```python
from build123d import *

# Parameters (mm, degrees)
BOSS_EXTRUDE1_DEPTH      = 2
CIRPATTERN1_COUNT        = 11
BOSS_EXTRUDE2_DEPTH      = 2
BOSS_EXTRUDE2_DEPTH_BACK = 2
SKETCH4_R                = 17.5
SKETCH6_R                = 14.669
SKETCH6_R_2              = 12.669
BOSS_EXTRUDE4_DEPTH      = 0.5
SKETCH7_R                = 10
CUT_EXTRUDE1_DEPTH       = 4
SKETCH8_W                = 2
SKETCH8_H                = 1.2
BOSS_EXTRUDE5_DEPTH      = 4
CIRPATTERN2_COUNT        = 12


with BuildPart() as part:
    # Sketch2 → Boss-Extrude1 (new, symmetric)
    with BuildSketch(Plane.XY):
        with BuildLine():
            Line((-0.5, 23.626113967), (0.5, 23.626113967))
            ThreePointArc((0.5, 23.626113967), (1.603484659, 21.216683922), (2.671054487, 18.791127038))
            ThreePointArc((2.671054487, 18.791127038), (3.577591086, 17.539110484), (4.930319745, 16.791127038))
            ThreePointArc((4.930319745, 16.791127038), (0, 17.5), (-4.930319745, 16.791127038))
            ThreePointArc((-4.930319745, 16.791127038), (-3.577591086, 17.539110484), (-2.671054487, 18.791127038))
            ThreePointArc((-2.671054487, 18.791127038), (-1.603484659, 21.216683922), (-0.5, 23.626113967))
        make_face()
    extrude(amount=BOSS_EXTRUDE1_DEPTH, both=True)


with BuildPart() as cirpattern1_1:
    # CirPattern1: pattern copy
    add(part.part.rotate(Axis((0, 0, 0), (0, 0, 1)), 1 * 360 / CIRPATTERN1_COUNT))


with BuildPart() as cirpattern1_2:
    # CirPattern1: pattern copy
    add(part.part.rotate(Axis((0, 0, 0), (0, 0, 1)), 2 * 360 / CIRPATTERN1_COUNT))


with BuildPart() as cirpattern1_3:
    # CirPattern1: pattern copy
    add(part.part.rotate(Axis((0, 0, 0), (0, 0, 1)), 3 * 360 / CIRPATTERN1_COUNT))


with BuildPart() as cirpattern1_4:
    # CirPattern1: pattern copy
    add(part.part.rotate(Axis((0, 0, 0), (0, 0, 1)), 4 * 360 / CIRPATTERN1_COUNT))


with BuildPart() as cirpattern1_5:
    # CirPattern1: pattern copy
    add(part.part.rotate(Axis((0, 0, 0), (0, 0, 1)), 5 * 360 / CIRPATTERN1_COUNT))


with BuildPart() as cirpattern1_6:
    # CirPattern1: pattern copy
    add(part.part.rotate(Axis((0, 0, 0), (0, 0, 1)), 6 * 360 / CIRPATTERN1_COUNT))


with BuildPart() as cirpattern1_7:
    # CirPattern1: pattern copy
    add(part.part.rotate(Axis((0, 0, 0), (0, 0, 1)), 7 * 360 / CIRPATTERN1_COUNT))


with BuildPart() as cirpattern1_8:
    # CirPattern1: pattern copy
    add(part.part.rotate(Axis((0, 0, 0), (0, 0, 1)), 8 * 360 / CIRPATTERN1_COUNT))


with BuildPart() as cirpattern1_9:
    # CirPattern1: pattern copy
    add(part.part.rotate(Axis((0, 0, 0), (0, 0, 1)), 9 * 360 / CIRPATTERN1_COUNT))


with BuildPart() as cirpattern1_10:
    # CirPattern1: pattern copy
    add(part.part.rotate(Axis((0, 0, 0), (0, 0, 1)), 10 * 360 / CIRPATTERN1_COUNT))


with BuildPart() as part_1:
    add(part.part)

    add(cirpattern1_1.part)  # Boss-Extrude2 merges CirPattern1_1

    add(cirpattern1_2.part)  # Boss-Extrude2 merges CirPattern1_2

    add(cirpattern1_3.part)  # Boss-Extrude2 merges CirPattern1_3

    add(cirpattern1_4.part)  # Boss-Extrude2 merges CirPattern1_4

    add(cirpattern1_5.part)  # Boss-Extrude2 merges CirPattern1_5

    add(cirpattern1_6.part)  # Boss-Extrude2 merges CirPattern1_6

    add(cirpattern1_7.part)  # Boss-Extrude2 merges CirPattern1_7

    add(cirpattern1_8.part)  # Boss-Extrude2 merges CirPattern1_8

    add(cirpattern1_9.part)  # Boss-Extrude2 merges CirPattern1_9

    add(cirpattern1_10.part)  # Boss-Extrude2 merges CirPattern1_10
    # Sketch4 → Boss-Extrude2 (add, two sides: drawn at the far end of the back side and taken through both)
    with BuildSketch(Plane.XY.offset(-BOSS_EXTRUDE2_DEPTH_BACK)):
        Circle(SKETCH4_R)
    extrude(amount=BOSS_EXTRUDE2_DEPTH + BOSS_EXTRUDE2_DEPTH_BACK)

    # Sketch6 → Boss-Extrude4 (add)
    with BuildSketch(Plane.XY.offset(2)):
        with Locations(Location((0, 0, 0), (0, 0, 180))):
            Circle(SKETCH6_R)
        Circle(SKETCH6_R_2, mode=Mode.SUBTRACT)
    extrude(amount=BOSS_EXTRUDE4_DEPTH)

    # Sketch7 → Cut-Extrude1 (cut)
    with BuildSketch(Plane.XY.offset(2)):
        Circle(SKETCH7_R)
    extrude(amount=-CUT_EXTRUDE1_DEPTH, mode=Mode.SUBTRACT)

    # Sketch8 → Boss-Extrude5 (add)
    with BuildSketch(Plane.XY.offset(2)):
        with Locations((0, 9.4)):
            Rectangle(SKETCH8_W, SKETCH8_H)
    boss_extrude5 = extrude(amount=-BOSS_EXTRUDE5_DEPTH)

    # CirPattern2: Boss-Extrude5 ×12 about axis
    cirpattern2_axis = Axis((0, 0, 0), (0, 0, 1))
    for i in range(1, CIRPATTERN2_COUNT):
        add(boss_extrude5.rotate(cirpattern2_axis, i * 360 / CIRPATTERN2_COUNT))


solid = part_1.part
```
Could you check a few things on this model? Use its own coordinates, in mm. A direction names the side the tool comes from. Coordinates: 2 decimals unless noted, no trailing zeros. Order: outer loops, then holes, each group sorted by start corner. A loop starts at its lowest first (then second) coordinate and runs counter-clockwise, first axis right, second up. Notation, with made-up numbers: M 78,-23 L 137,-23 A17 cw 137,-5 Z; hole C 22.5,-14.5 d9. An arc over 180 degrees is marked long. Use one line per item in the form item = value. Start each with the question number.
1. On a 3-axis mill with a long thin cutter (end or side, diameter ignored), from which of +Z, -Z, +X, -X, +Y, -Y can I reach the whole of each face in a straight line? I mean faces 1 (the flat face through (0, 23.626, 0)), 2 (the cylindrical face through (-2.746, -12.368, 2.246)), 3 (the flat face through (-3.817, -8.612, 0.028)). Say none if no direction works.
2. Suppose I cut it at B-B on y = -12. Write out the boundary of the cut face in (x, z).
3. Please list where these lines run through material, in increasing order: line 1 (Y direction, x = 0, z = 2.45); line 2 (X direction, y = 17, z = 0.95); line 3 (X direction, y = 17.5, z = 0).
4. For pin 1 (4 mm diameter, centred on x = 14.5, y = -7.5, fed in from +Z); pin 2 (1.3 mm diameter, centred on y = -9.5, z = 0, fed in from +X); pin 3 (0.9 mm diameter, centred on x = -9.5, z = -1, fed in from +Y); pin 4 (0.9 mm diameter, centred on y = -9.5, z = 0, fed in from -X), each with a flat end and sliding along its axis, tell me the tip position at first contact or that it passes through.
5. We'd pull the mould along Y, two halves only. Please class faces 4 (the flat face through (-8.612, -3.817, 0.028)), 5 (the cylindrical face through (4.463, -20.837, 0.028)), 6 (the flat face through (13, 0, 2.5)), 7 (the cylindrical face through (1.59, 21.25, 0.03)): +Y half, -Y half, draft (parallel to the pull), parting line (faces both ways), or undercut.
6. Suppose I cut it at A-A on x = 14. Write out the boundary of the cut face in (y, z).
7. Suppose I cut it at C-C on y = 16. Write out the boundary of the cut face in (x, z).
Geometry says:
q1.face_1 = +Z, -Z, +X, -X, +Y
q1.face_2 = +Z
q1.face_3 = +Z, -Z
q2.outline = M -16.77,-2 L 16.77,-2 L 16.77,2 L 8.44,2 L 8.44,2.5 L 4.06,2.5 L 4.06,2 L -4.06,2 L -4.06,2.5 L -8.44,2.5 L -8.44,2 L -16.77,2 Z
q3.line_1 = -14.67 to -12.67, 12.67 to 14.67
q3.line_2 = -12.82 to -7.47, -4.39 to 4.39, 7.47 to 12.82
q3.line_3 = -12.9 to -8.28, -3.62 to 3.62, 8.28 to 12.9
q4.pin_1 = 2.5
q4.pin_2 = 15.89
q4.pin_3 = 18.6
q4.pin_4 = -15.81
q5.face_4 = undercut
q5.face_5 = -Y half
q5.face_6 = draft
q5.face_7 = +Y half
q6.outline = M -14.81,-2 L 10.79,-2 L 10.79,2 L 4.38,2 L 4.38,2.5 L -4.38,2.5 L -4.38,2 L -14.81,2 Z
q7.outline = M -12.67,-2 L 12.67,-2 L 12.67,2 L -12.67,2 Z
